The model under review builds one solid part; all positions refer to its coordinate system, in mm. Face numbers are marked on the shaded views. A direction names the side the tool comes from. Give positions to 0.01 mm unless a question says otherwise; leave off trailing zeros. Order: outer loops, then holes, each group sorted by start corner. A loop starts at its lowest first (then second) coordinate and runs counter-clockwise, first axis right, second up. Notation, with made-up numbers: (-38.75, -20.5) - (-29.75, -20.5) arc R13 ccw to (-29.75, 4.5) - close; hole circle Ø8 at (85, 53.5). An arc over 180 degrees is marked (long way). Use CSV: the item, a comma, the result in double quotes.
```python
from build123d import *

# Parameters (mm, degrees)
BOX008_W           = 4
BOX008_H           = 1
BOX008_DEPTH       = 7
BOX010_W           = 4
BOX010_H           = 1
BOX010_DEPTH       = 7
BOX007_W           = 4
BOX007_H           = 2
BOX007_DEPTH       = 7
BOX009_W           = 4
BOX009_H           = 1
BOX009_DEPTH       = 7
BOX006_W           = 4
BOX006_H           = 1
BOX006_DEPTH       = 7
BOX011_W           = 4
BOX011_H           = 7.2
BOX011_DEPTH       = 7
BOX005_W           = 13
BOX005_H           = 40
BOX005_DEPTH       = 10
BOX005_PITCH_ANGLE = -45
BOX_W              = 10
BOX_H              = 2
BOX_DEPTH          = 7
BOX002_W           = 10
BOX002_H           = 2
BOX002_DEPTH       = 7
BOX003_W           = 10
BOX003_H           = 2
BOX003_DEPTH       = 7
BOX004_W           = 10
BOX004_H           = 2
BOX004_DEPTH       = 7
BOX001_W           = 5
BOX001_H           = 40
BOX001_DEPTH       = 7
CHAMFER_SIZE       = 4


with BuildPart() as cube008:
    # Box008 → Box008 (new body)
    with BuildSketch(Plane(origin=(-1, 12, 0), x_dir=(1, 0, 0), z_dir=(0, 0, 1))):
        with Locations((2, 0.5)):
            Rectangle(BOX008_W, BOX008_H)
    extrude(amount=BOX008_DEPTH)


with BuildPart() as cube010:
    # Box010 → Box010 (new body)
    with BuildSketch(Plane(origin=(-1, 36.6, 0), x_dir=(1, 0, 0), z_dir=(0, 0, 1))):
        with Locations((2, 0.5)):
            Rectangle(BOX010_W, BOX010_H)
    extrude(amount=BOX010_DEPTH)


with BuildPart() as cube007:
    # Box007 → Box007 (new body)
    with BuildSketch(Plane(origin=(-1, 8, 0), x_dir=(1, 0, 0), z_dir=(0, 0, 1))):
        with Locations((2, 1)):
            Rectangle(BOX007_W, BOX007_H)
    extrude(amount=BOX007_DEPTH)


with BuildPart() as cube009:
    # Box009 → Box009 (new body)
    with BuildSketch(Plane(origin=(-1, 24.4, 0), x_dir=(1, 0, 0), z_dir=(0, 0, 1))):
        with Locations((2, 0.5)):
            Rectangle(BOX009_W, BOX009_H)
    extrude(amount=BOX009_DEPTH)


with BuildPart() as cube006:
    # Box006 → Box006 (new body)
    with BuildSketch(Plane(origin=(-1, 5, 0), x_dir=(1, 0, 0), z_dir=(0, 0, 1))):
        with Locations((2, 0.5)):
            Rectangle(BOX006_W, BOX006_H)
    extrude(amount=BOX006_DEPTH)


with BuildPart() as fusion003:
    # Box011 → Box011 (new body)
    with BuildSketch(Plane(origin=(-1, 27.4, 0), x_dir=(1, 0, 0), z_dir=(0, 0, 1))):
        with Locations((2, 3.6)):
            Rectangle(BOX011_W, BOX011_H)
    extrude(amount=BOX011_DEPTH)

    # Fusion003: union Cube008, Cube010, Cube007, Cube009, Cube006
    add(cube008.part)
    add(cube010.part)
    add(cube007.part)
    add(cube009.part)
    add(cube006.part)


with BuildPart() as sphere010:
    # Sphere010 → Sphere010 (revolve)
    with BuildSketch(Plane(origin=(-3, 28, 2.5), x_dir=(1, 0, 0), z_dir=(0, -1, 0))):
        with BuildLine():
            ThreePointArc((0, -1.5), (1.5, 0), (0, 1.5))
            Line((0, 1.5), (0, -1.5))
        make_face()
    revolve(axis=Axis((-3, 28, 2.5), (0, 0, 1)))


with BuildPart() as fusion002:
    # Sphere011 → Sphere011 (revolve)
    with BuildSketch(Plane(origin=(-3, 34, 2.5), x_dir=(1, 0, 0), z_dir=(0, -1, 0))):
        with BuildLine():
            ThreePointArc((0, -1.5), (1.5, 0), (0, 1.5))
            Line((0, 1.5), (0, -1.5))
        make_face()
    revolve(axis=Axis((-3, 34, 2.5), (0, 0, 1)))

    # Fusion002: union Sphere010
    add(sphere010.part)


with BuildPart() as sphere009:
    # Sphere009 → Sphere009 (revolve)
    with BuildSketch(Plane(origin=(-3, 11.5, 2.5), x_dir=(1, 0, 0), z_dir=(0, -1, 0))):
        with BuildLine():
            ThreePointArc((0, -1.25), (1.25, 0), (0, 1.25))
            Line((0, 1.25), (0, -1.25))
        make_face()
    revolve(axis=Axis((-3, 11.5, 2.5), (0, 0, 1)))


with BuildPart() as cube005:
    # Box005 → Box005 (new body)
    with BuildSketch(Plane.XY):
        with Locations((6.5, 20)):
            Rectangle(BOX005_W, BOX005_H)
    extrude(amount=BOX005_DEPTH)


with BuildPart() as cube005_1:
    # Box005 pitch: moved
    add(cube005.part.rotate(Axis((0, 0, 0), (0, 1, 0)), BOX005_PITCH_ANGLE))


with BuildPart() as cube005_2:
    # Box005 placement: moved
    add(cube005_1.part.moved(Location((-10.19, 0, -1.19))))


with BuildPart() as cube:
    # Box → Box (new body)
    with BuildSketch(Plane(origin=(-10, 6, 0), x_dir=(1, 0, 0), z_dir=(0, 0, 1))):
        with Locations((5, 1)):
            Rectangle(BOX_W, BOX_H)
    extrude(amount=BOX_DEPTH)


with BuildPart() as cube002:
    # Box002 → Box002 (new body)
    with BuildSketch(Plane(origin=(-10, 10, 0), x_dir=(1, 0, 0), z_dir=(0, 0, 1))):
        with Locations((5, 1)):
            Rectangle(BOX002_W, BOX002_H)
    extrude(amount=BOX002_DEPTH)


with BuildPart() as cube003:
    # Box003 → Box003 (new body)
    with BuildSketch(Plane(origin=(-10, 25.4, 0), x_dir=(1, 0, 0), z_dir=(0, 0, 1))):
        with Locations((5, 1)):
            Rectangle(BOX003_W, BOX003_H)
    extrude(amount=BOX003_DEPTH)


with BuildPart() as cube004:
    # Box004 → Box004 (new body)
    with BuildSketch(Plane(origin=(-10, 34.6, 0), x_dir=(1, 0, 0), z_dir=(0, 0, 1))):
        with Locations((5, 1)):
            Rectangle(BOX004_W, BOX004_H)
    extrude(amount=BOX004_DEPTH)


with BuildPart() as cut:
    # Box001 → Box001 (new body)
    with BuildSketch(Plane.XY):
        with Locations((2.5, 20)):
            Rectangle(BOX001_W, BOX001_H)
    extrude(amount=BOX001_DEPTH)

    # Fusion: union Cube, Cube002, Cube003, Cube004
    add(cube.part)
    add(cube002.part)
    add(cube003.part)
    add(cube004.part)

    # Cut: cut Cube005
    add(cube005_2.part, mode=Mode.SUBTRACT)


with BuildPart() as cut002:
    # Sphere008 → Sphere008 (revolve)
    with BuildSketch(Plane(origin=(-3, 6.5, 2.5), x_dir=(1, 0, 0), z_dir=(0, -1, 0))):
        with BuildLine():
            ThreePointArc((0, -1.25), (1.25, 0), (0, 1.25))
            Line((0, 1.25), (0, -1.25))
        make_face()
    revolve(axis=Axis((-3, 6.5, 2.5), (0, 0, 1)))

    # Fusion001: union Sphere009, Cut
    add(sphere009.part)
    add(cut.part)

    # Cut001: cut Fusion002
    add(fusion002.part, mode=Mode.SUBTRACT)

    # Chamfer
    chamfer_edges = [cut002.edges().sort_by_distance(p)[0] for p in [
        (-9, 7, 0),
        (-9, 11, 0),
        (-9, 35.6, 0),
        (-9, 26.4, 0),
    ]]
    chamfer(chamfer_edges, length=CHAMFER_SIZE)

    # Cut002: cut Fusion003
    add(fusion003.part, mode=Mode.SUBTRACT)


solid = cut002.part
```
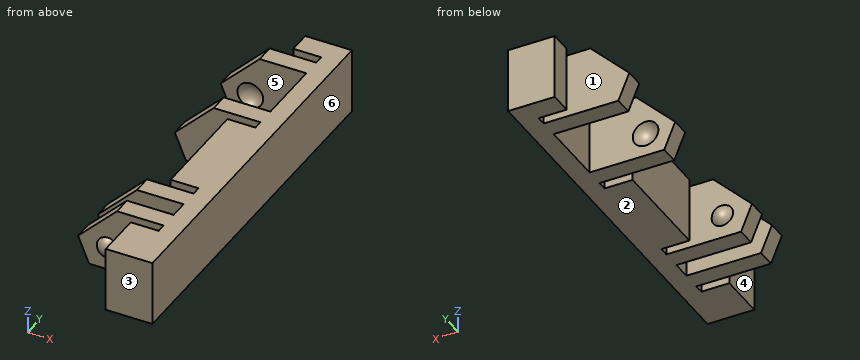
Item 1: Clearance check with flat-ended pins moving along their axes: pin 1 (2 mm diameter, centred on y = 33, z = 5, fed in from -X); pin 2 (3.5 mm diameter, centred on x = -3, z = 4, fed in from +Y); pin 3 (1 mm diameter, centred on x = -2.5, z = 4.5, fed in from -Y). State where each tip first meets the part, or that it passes through.
Results list:
pin 1,"stops at x = 3"
pin 2,"stops at y = 36.6"
pin 3,"stops at y = 6"
Item 2: Take a section at C-C, the plane y = 25. Give the boundary of the cut face in (x, z).
Results list:
outline,"(3, 0) - (5, 0) - (5, 7) - (3, 7) - close"
Item 3: Wall thickness on L1, parallel to Y at x = -2.75, z = 5.5; L2, parallel to Y at x = -3.25, z = 2.25; L3, parallel to X at y = 9, z = 5: over which ranges is each line inside the solid? List them lowest first.
Results list:
L1,"y = 6 to 8, 10 to 12, 25.4 to 27.4, 34.6 to 36.6"
L2,"y = 5.3 to 8, 10 to 12.7, 25.4 to 26.54, 35.46 to 36.6"
L3,"x = 3 to 5"
Item 4: Take a section at A-A, the plane x = 1.75. Give the boundary of the cut face in (y, z).
Results list:
outline,"(0, 0) - (5, 0) - (5, 7) - (0, 7) - close; (6, 0) - (8, 0) - (8, 7) - (6, 7) - close; (10, 0) - (12, 0) - (12, 7) - (10, 7) - close; (13, 0) - (24.4, 0) - (24.4, 7) - (13, 7) - close; (25.4, 0) - (27.4, 0) - (27.4, 7) - (25.4, 7) - close; (34.6, 0) - (36.6, 0) - (36.6, 7) - (34.6, 7) - close; (37.6, 0) - (40, 0) - (40, 7) - (37.6, 7) - close"
Item 5: Take a section at B-B, the plane x = -0.5. Give the boundary of the cut face in (y, z), and give its area (3 significant figures).
Results list:
outline,"(6, 0) - (8, 0) - (8, 7) - (6, 7) - close; (10, 0) - (12, 0) - (12, 7) - (10, 7) - close; (25.4, 0) - (27.4, 0) - (27.4, 7) - (25.4, 7) - close; (34.6, 0) - (36.6, 0) - (36.6, 7) - (34.6, 7) - close"
area,"56.0 mm2"
Item 6: Take a section at D-D, the plane x = -3.75. Give the boundary of the cut face in (y, z).
Results list:
outline,"(6, 0) - (8, 0) - (8, 5.25) - (6, 5.25) - (6, 3.37) arc R1 ccw to (6, 1.63) - close; (10, 0) - (12, 0) - (12, 1.63) arc R1 ccw to (12, 3.37) - (12, 5.25) - (10, 5.25) - close; (25.4, 0) - (27.4, 0) - (27.4, 1.35) arc R1.3 cw to (27.4, 3.65) - (27.4, 5.25) - (25.4, 5.25) - close; (34.6, 0) - (36.6, 0) - (36.6, 5.25) - (34.6, 5.25) - (34.6, 3.65) arc R1.3 cw to (34.6, 1.35) - close"
Item 7: Tool access review of the marked faces 4, 5 and 6: name each direction out of +Z, -Z, +X, -X, +Y, -Y from which nothing blocks a thin tool from reaching the whole face with its end or side.
Results list:
face 4,"+Z, -Z, -X, -Y"
face 5,"+Z, -Z, -X"
face 6,"+Z, -Z, +X, +Y, -Y"
Item 8: Mouldability with a two-part tool opening along Y and no side actions: class the marked faces 1, 2 and 3 as pulls with the +Y half, pulls with the -Y half, needs draft (parallel to the pull), parting line crosses it, or undercut.
Results list:
face 1,"undercut"
face 2,"needs draft"
face 3,"pulls with the -Y half"
